```python
from build123d import *

# Parameters (mm, degrees)
SKETCH026_R     = 4
PAD015_DEPTH    = 110
SKETCH027_R     = 11.25
PAD016_DEPTH    = 75
SKETCH029_R     = 8
PAD017_DEPTH    = 90
POCKET012_DEPTH = 18


with BuildPart() as part:
    # Sketch026 → Pad015 (new body)
    with BuildSketch(Plane.YZ):
        Circle(SKETCH026_R)
    extrude(amount=-PAD015_DEPTH)

    # Sketch027 → Pad016 (new body, symmetric)
    with BuildSketch(Plane.YZ):
        Circle(SKETCH027_R)
    extrude(amount=PAD016_DEPTH, both=True)

    # Sketch029 → Pad017 (new body)
    with BuildSketch(Plane.YZ):
        Circle(SKETCH029_R)
    extrude(amount=PAD017_DEPTH)

    # Sketch028 → Pocket012 (cut)
    with BuildSketch(Plane.YZ.offset(90)):
        with BuildLine():
            ThreePointArc((2.99806, -0.107877), (-1.918287, 2.306551), (-0.44036, -2.967505))
            Line((-0.44036, -2.967505), (0.198883, -3.73651))
            Line((0.198883, -3.73651), (3.637995, -0.877715))
            Line((2.99806, -0.107877), (3.637995, -0.877715))
        make_face()
    extrude(amount=-POCKET012_DEPTH, mode=Mode.SUBTRACT)


solid = part.part
```
Verification items for the finished model (mm, model axes). A direction names the side the tool comes from. Give positions to 0.01 mm unless a question says otherwise; leave off trailing zeros. Order: outer loops, then holes, each group sorted by start corner. A loop starts at its lowest first (then second) coordinate and runs counter-clockwise, first axis right, second up. Notation, with made-up numbers: (74, 26.5) -> (114, 26.5) arc R27 ccw to (114, 59.5) -> close; hole circle Ø2 at (-27, 23.25). An arc over 180 degrees is marked (long way). Use a Markdown table: item, result.
1) Tool access check on faces 1 (the flat face through (90, 3.4, 0.1)), 2 (the cylindrical face through (82.4, -1.73, -7.81)), 3 (the flat face through (-75, 5, 0)). Record the directions out of +Z, -Z, +X, -X, +Y, -Y that give a thin tool (end or side, any length) a straight path to the whole face; none if there is none.
Results:
| item | result |
|---|---|
| face 1 | +Z, -Z, +X, +Y, -Y |
| face 2 | +X |
| face 3 | -X |
2) Section check A-A, the plane x = -22.5. Record the boundary of the cut face in (y, z), then the cut area to 3 significant figures.
Results:
| item | result |
|---|---|
| outline | circle Ø22.5 at (0, 0) |
| area | 398 mm² |
3) Mould release check, pull along Y, two halves, no side actions. Record for faces 4 (the cylindrical face through (81.1, -1.8, 2.4)), 5 (the flat face through (75, 2, 8)), 6 (the cylindrical face through (-92.255, -0.867, -3.905)): pulls with the +Y half, pulls with the -Y half, needs draft (parallel to the pull), parting line crosses it, or undercut.
Results:
| item | result |
|---|---|
| face 4 | undercut |
| face 5 | needs draft |
| face 6 | parting line crosses it |
4) Material ranges on probe 1 along Y at (x, z) = (81.5, 0); probe 2 along X at (y, z) = (-5.75, 5.25); probe 3 along Z at (x, y) = (79.75, 0), recorded low to high.
Results:
| item | result |
|---|---|
| probe 1 | -8 to -3, 3 to 8 |
| probe 2 | -75 to 90 |
| probe 3 | -8 to -3.5, 3 to 8 |
5) Depth check by flat-ended pin: pin 1 Ø8 at (x, z) = (-51, 3.5) entering from +Y; pin 2 Ø8 at (x, z) = (22.5, -4.5) entering from -Y; pin 3 Ø6 at (x, z) = (27.5, 6.5) entering from +Y; pin 4 Ø1.5 at (x, z) = (-3, 6) entering from -Y. Enter the tip coordinate at first touch or a pass-through.
Results:
| item | result |
|---|---|
| pin 1 | y = 11.25 |
| pin 2 | y = -11.24 |
| pin 3 | y = 10.69 |
| pin 4 | y = -9.95 |
